Geometry: final body of the model. Coordinates: model frame, mm. Give positions to 0.01 mm unless a question says otherwise; leave off trailing zeros. Write each loop counter-clockwise with the first axis right and the second up, starting at its lowest first coordinate (ties: lowest second). Pieces come first, ordered by that corner, then holes. Notation, with made-up numbers: M -9,72 L 40,72 A19 ccw 40,104 Z; hole C -2,55.5 d4. An arc over 180 degrees is marked long. Use a Markdown table: item, result. Add a question column.
(1) Cut plane D-D (y = 40). Output: boundary loops of the cut face in (x, z), plus the area to 3 significant figures.
(2) Cut plane B-B (y = -30). Output: boundary loops of the cut face in (x, z), plus the area to 3 significant figures.
(3) Cut plane A-A (z = 0). Output: boundary loops of the cut face in (x, y), plus the area to 3 significant figures.
(4) Cut plane C-C (x = 0). Output: boundary loops of the cut face in (y, z), plus the area to 3 significant figures.
(5) Material intervals for L1, parallel to Y at x = 0, z = -3.5; L2, parallel to Y at x = -0.25, z = 0; L3, parallel to Y at x = 5.5, z = 0, sorted ascending.
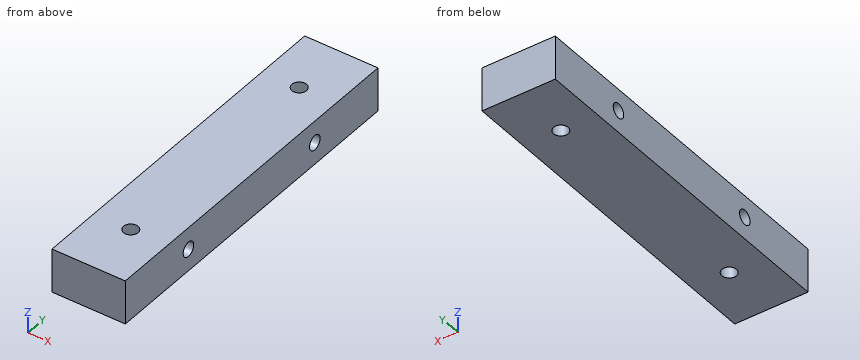
```python
from build123d import *

# Parameters (mm, degrees)
SKETCH1_W           = 25
SKETCH1_H           = 15
BOSS_EXTRUDE1_DEPTH = 60
M6_TAPPED_HOLE1_D   = 5
M6_TAPPED_HOLE2_D   = 5


with BuildPart() as part:
    # Sketch1 → Boss-Extrude1 (new body, symmetric)
    with BuildSketch(Plane(origin=(0, 0, 0), x_dir=(1, 0, 0), z_dir=(0, 1, 0))):
        Rectangle(SKETCH1_W, SKETCH1_H)
    extrude(amount=BOSS_EXTRUDE1_DEPTH, both=True)

    # M6 Tapped Hole1 (through all)
    with Locations(Plane.ZY.offset(12.5)):
        with Locations((0, 30), (0, -30)):
            Hole(M6_TAPPED_HOLE1_D / 2)

    # M6 Tapped Hole2 (through all)
    with Locations(Plane.XY.offset(7.5)):
        with Locations((0, 40), (0, -40)):
            Hole(M6_TAPPED_HOLE2_D / 2)


solid = part.part
```
Answer list:
| question | item | result |
|---|---|---|
| 1 | outline | M -12.5,-7.5 L -2.5,-7.5 L -2.5,7.5 L -12.5,7.5 Z; M 2.5,-7.5 L 12.5,-7.5 L 12.5,7.5 L 2.5,7.5 Z |
| 1 | area | 300 mm² |
| 2 | outline | M -12.5,-7.5 L 12.5,-7.5 L 12.5,-2.5 L -12.5,-2.5 Z; M -12.5,2.5 L 12.5,2.5 L 12.5,7.5 L -12.5,7.5 Z |
| 2 | area | 250 mm² |
| 3 | outline | M -12.5,-60 L 12.5,-60 L 12.5,-32.5 L -12.5,-32.5 Z; M -12.5,-27.5 L 12.5,-27.5 L 12.5,27.5 L -12.5,27.5 Z; M -12.5,32.5 L 12.5,32.5 L 12.5,60 L -12.5,60 Z; hole C 0,-40 d5; hole C 0,40 d5 |
| 3 | area | 2,710 mm² |
| 4 | outline | M -60,-7.5 L -42.5,-7.5 L -42.5,7.5 L -60,7.5 Z; M -37.5,-7.5 L 37.5,-7.5 L 37.5,7.5 L -37.5,7.5 Z; M 42.5,-7.5 L 60,-7.5 L 60,7.5 L 42.5,7.5 Z; hole C -30,0 d5; hole C 30,0 d5 |
| 4 | area | 1,610 mm² |
| 5 | L1 | -60 to -42.5, -37.5 to 37.5, 42.5 to 60 |
| 5 | L2 | -60 to -42.49, -37.51 to -32.5, -27.5 to 27.5, 32.5 to 37.51, 42.49 to 60 |
| 5 | L3 | -60 to -32.5, -27.5 to 27.5, 32.5 to 60 |
